Model file for the job. Use its own axes, mm. Face numbers are marked on the shaded views. A direction names the side the tool comes from. Coordinates: 2 decimals unless noted, no trailing zeros. Write each loop counter-clockwise with the first axis right and the second up, starting at its lowest first coordinate (ties: lowest second). Pieces come first, ordered by that corner, then holes. Notation, with made-up numbers: M -11.75,-17.75 L 3.25,-17.75 A4 cw 3.25,-12.75 Z; hole C 0.25,-40 d7. An arc over 180 degrees is marked long. Answer in a Markdown table with one row per item. Add a question column.
```python
from build123d import *

# Parameters (mm, degrees)
SKETCH1_R           = 5
BOSS_EXTRUDE1_DEPTH = 27.5
SKETCH2_R           = 6.25
BOSS_EXTRUDE2_DEPTH = 3
SKETCH3_R           = 4
BOSS_EXTRUDE3_DEPTH = 3.5
CHAMFER1_SIZE       = 3
CHAMFER1_SIZE_2     = 1
FILLET1_R           = 0.3
FILLET2_R           = 0.15


with BuildPart() as part:
    # Sketch1 → Boss-Extrude1 (new body)
    with BuildSketch(Plane(origin=(0, 0, 0), x_dir=(1, 0, 0), z_dir=(0, 1, 0))):
        with Locations(Location((0, 0, 0), (0, 0, 270))):
            Circle(SKETCH1_R)
    extrude(amount=BOSS_EXTRUDE1_DEPTH)

    # Sketch2 → Boss-Extrude2 (add)
    with BuildSketch(Plane(origin=(0, 27.5, 0), x_dir=(1, 0, 0), z_dir=(0, 1, 0))):
        with Locations(Location((0, 0, 0), (0, 0, 270))):
            Circle(SKETCH2_R)
    extrude(amount=BOSS_EXTRUDE2_DEPTH)

    # Sketch3 → Boss-Extrude3 (add)
    with BuildSketch(Plane(origin=(0, 30.5, 0), x_dir=(1, 0, 0), z_dir=(0, 1, 0))):
        with Locations(Location((0, 0, 0), (0, 0, 270))):
            Circle(SKETCH3_R)
    extrude(amount=BOSS_EXTRUDE3_DEPTH)

    # Chamfer1
    # the kernel refuses this chamfer: 3, 1 mm, written as the material it takes off along each edge
    with BuildSketch(Plane(origin=(0, 30.5, 0), x_dir=(0, 0, 1), z_dir=(-1, 0, 0))) as chamfer1_piece_1:
        Polygon((6.25, -CHAMFER1_SIZE), (6.25 - CHAMFER1_SIZE_2, 0), (6.25, 0), align=None)
    revolve(axis=Axis((0, 30.5, 0), (0, 1, 0)), mode=Mode.SUBTRACT)

    # Fillet1
    fillet1_edges = [part.edges().sort_by_distance(p)[0] for p in [
        (0, 34, -4),
    ]]
    fillet(fillet1_edges, radius=FILLET1_R)

    # Fillet2
    fillet2_edges = [part.edges().sort_by_distance(p)[0] for p in [
        (0, 30.5, -5.25),
    ]]
    fillet(fillet2_edges, radius=FILLET2_R)


solid = part.part
```
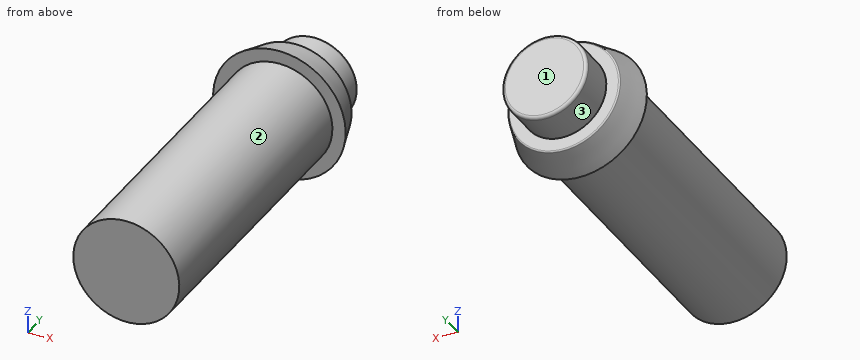
1) Slice it at C-C (y = 5). Give the cut face in (x, z), then the cut area to 3 significant figures.
2) Flat gauge pins, fed straight in: pin 1 Ø1.5 at (x, y) = (-2.5, 30) entering from +Z; pin 2 Ø4 at (x, z) = (-5, -4.5) entering from +Y; pin 3 Ø4 at (x, y) = (2, 15) entering from +Z. Where does each tip first touch, or does it go through?
3) Slice it at B-B (z = 0). Give the cut face in (x, y).
4) Drill centre lines: probe 1 along Y at (x, z) = (2.25, 3.5); probe 2 along Y at (x, z) = (-5, -1); probe 3 along X at (y, z) = (20.5, 0.25). Where is each one in solid material? Low to high.
5) Which spindle directions (+Z, -Z, +X, -X, +Y, -Y) get a long thin tool onto all of the face, cutting with end or side? Do the marked faces 1, 2 and 3. Say none if no direction does.
6) Slice it at A-A (x = 0). Give the cut face in (y, z).
Ans:
| question | item | result |
|---|---|---|
| 1 | outline | C 0,0 d10 |
| 1 | area | 78.5 mm2 |
| 2 | pin 1 | stops at z = 5.24 |
| 2 | pin 2 | stops at y = 30.5 |
| 2 | pin 3 | stops at z = 5 |
| 3 | outline | M -6.25,27.5 L -5,27.5 L -5,0 L 5,0 L 5,27.5 L 6.25,27.5 L 5.28,30.4 A0.15 ccw 5.14,30.5 L 4,30.5 L 4,33.7 A0.3 ccw 3.7,34 L -3.7,34 A0.3 ccw -4,33.7 L -4,30.5 L -5.14,30.5 A0.15 ccw -5.28,30.4 Z |
| 4 | probe 1 | y = 0 to 30.5 |
| 4 | probe 2 | y = 27.5 to 30.5 |
| 4 | probe 3 | x = -4.99 to 4.99 |
| 5 | face 1 | +Z, -Z, +X, -X, +Y |
| 5 | face 2 | -Y |
| 5 | face 3 | +Y |
| 6 | outline | M 0,-5 L 27.5,-5 L 27.5,-6.25 L 30.4,-5.28 A0.15 ccw 30.5,-5.14 L 30.5,-4 L 33.7,-4 A0.3 ccw 34,-3.7 L 34,3.7 A0.3 ccw 33.7,4 L 30.5,4 L 30.5,5.14 A0.15 ccw 30.4,5.28 L 27.5,6.25 L 27.5,5 L 0,5 Z |
